The figure shows three views and two pictorial views of one solid part (mm, origin at its lowest corner). Answer the questions. Give positions to 0.01 mm unless a question says otherwise; leave off trailing zeros. Order: outer loops, then holes, each group sorted by start corner. A loop starts at its lowest first (then second) coordinate and runs counter-clockwise, first axis right, second up. Notation, with made-up numbers: M 54,-22.75 L 97,-22.75 A4 ccw 97,-15.75 Z; hole C -34,23 d11. An arc over 180 degrees is marked long. One line per item, written item: value.
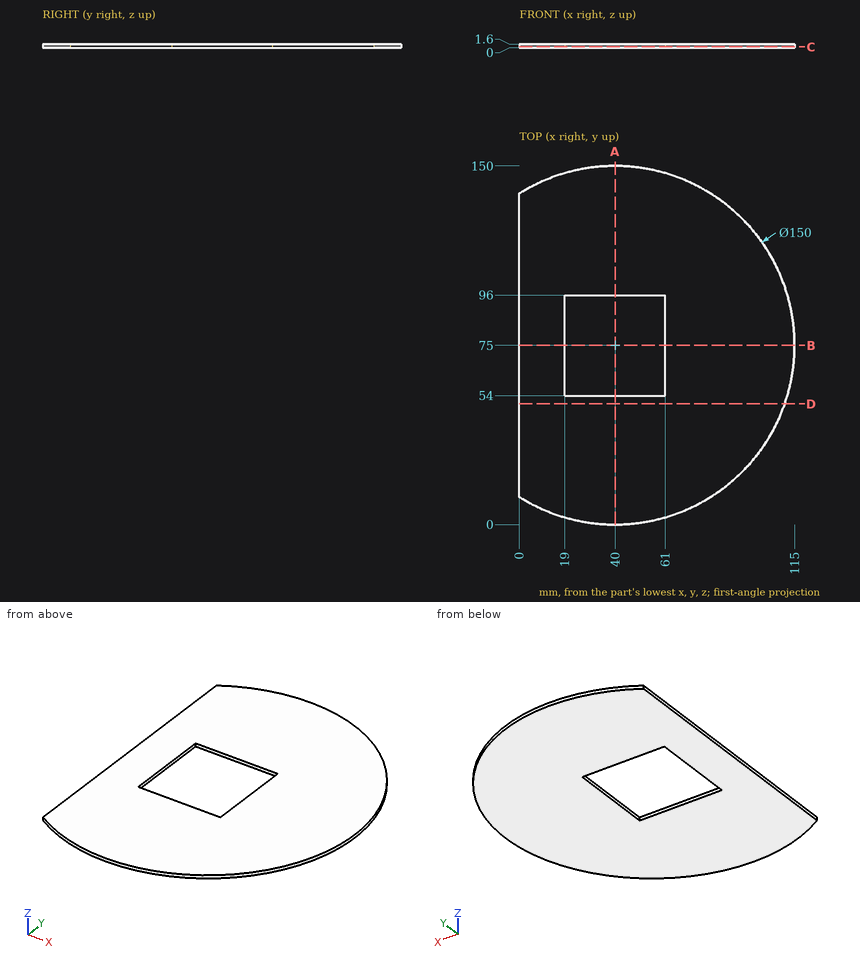
1) Find section B-B, the plane y = 75. Write down the section's boundary in (x, z).
Reported:
outline: M 0,0 L 19,0 L 19,1.6 L 0,1.6 Z; M 61,0 L 115,0 L 115,1.6 L 61,1.6 Z
2) Find section C-C, the plane z = 0.4. Write down the section's boundary in (x, y), plus the area to 3 significant figures.
Reported:
outline: M 0,11.56 A75 ccw long 0,138.44 Z; hole M 19,54 L 61,54 L 61,96 L 19,96 Z
area: 12,800 mm^2
3) Consider probe 1 along Y at (x, z) = (42, 0.1); probe 2 along Y at (x, z) = (56, 1.05); probe 3 along X at (y, z) = (83, 1.05). Determine where each line is inside the solid, lowest interval first.
Reported:
probe 1: y = 0.03 to 54, 96 to 149.97
probe 2: y = 1.73 to 54, 96 to 148.27
probe 3: x = 0 to 19, 61 to 114.57
4) This flat-tipped pin is pushed along its axis until it touches: pin 1 Ø4 at (x, y) = (48.5, 33) entering from -Z. Where does it stop, or does it pass through?
Reported:
pin 1: stops at z = 0
5) Find section D-D, the plane y = 50.5. Write down the section's boundary in (x, z), plus the area to 3 significant figures.
Reported:
outline: M 0,0 L 110.89,0 L 110.89,1.6 L 0,1.6 Z
area: 177 mm^2
6) Find section A-A, the plane x = 40. Write down the section's boundary in (y, z).
Reported:
outline: M 0,0 L 54,0 L 54,1.6 L 0,1.6 Z; M 96,0 L 150,0 L 150,1.6 L 96,1.6 Z
